```python
from build123d import *

# Parameters (mm, degrees)
SKETCH_1_W      = 20
SKETCH_1_H      = 8
EXTRUDE_1_DEPTH = 5
SKETCH_5_W      = 5
SKETCH_5_H      = 5
EXTRUDE_5_DEPTH = 10
SKETCH_8_W      = 20
SKETCH_8_H      = 8
EXTRUDE_6_DEPTH = 55
EXTRUDE_6_TAPER = 1
SKETCH_9_W      = 5
SKETCH_9_H      = 5
EXTRUDE_7_DEPTH = 11
SKETCH_10_W     = 5
SKETCH_10_H     = 5
EXTRUDE_8_DEPTH = 11


with BuildPart() as part:
    # ｽｹｯﾁ1 → ﾎﾞｽ - 押し出し1 (new body)
    with BuildSketch(Plane.XY):
        Rectangle(SKETCH_1_W, SKETCH_1_H)
    extrude(amount=EXTRUDE_1_DEPTH)

    # ｽｹｯﾁ5 → ﾎﾞｽ - 押し出し5 (add)
    with BuildSketch(Plane(origin=(0, 0, 0), x_dir=(-1, 0, 0), z_dir=(0, 0, -1))):
        Rectangle(SKETCH_5_W, SKETCH_5_H)
    extrude(amount=EXTRUDE_5_DEPTH)

    # ｽｹｯﾁ8 → ﾎﾞｽ - 押し出し6 (add)
    with BuildSketch(Plane.XY.offset(5)):
        Rectangle(SKETCH_8_W, SKETCH_8_H)
    extrude(amount=EXTRUDE_6_DEPTH, taper=EXTRUDE_6_TAPER)

    # ｽｹｯﾁ9 → ﾎﾞｽ - 押し出し7 (add)
    with BuildSketch(Plane(origin=(0, 4, 0), x_dir=(1, 0, 0), z_dir=(0, 1, 0))):
        with Locations((0, -2.5)):
            Rectangle(SKETCH_9_W, SKETCH_9_H)
    extrude(amount=EXTRUDE_7_DEPTH)

    # ｽｹｯﾁ10 → ﾎﾞｽ - 押し出し8 (add)
    with BuildSketch(Plane(origin=(0, -4, 0), x_dir=(-1, 0, 0), z_dir=(0, -1, 0))):
        with Locations((0, -2.5)):
            Rectangle(SKETCH_10_W, SKETCH_10_H)
    extrude(amount=EXTRUDE_8_DEPTH)


solid = part.part
```
Geometry check sheet. Reference: the model listing, model coordinates, mm. A direction names the side the tool comes from. Coordinates: 2 decimals unless noted, no trailing zeros. Order: outer loops, then holes, each group sorted by start corner. A loop starts at its lowest first (then second) coordinate and runs counter-clockwise, first axis right, second up.
Q1. Tool access check on faces 1 (the face through (0, 9, 5)), 2 (the face through (-2.5, -9, 3)), 3 (the face through (2.5, -9, 3)), 4 (the face through (-2.5, 0, -5)), 5 (the face through (6, 4, 2)). Record the directions out of +Z, -Z, +X, -X, +Y, -Y that give a thin tool (end or side, any length) a straight path to the whole face; none if there is none.
Reply:
face 1: +Z, +X, -X, +Y
face 2: +Z, -Z, -X, -Y
face 3: +Z, -Z, +X, -Y
face 4: -Z, -X, +Y, -Y
face 5: +Z, -Z, +X, +Y
Q2. Sectioned sample at C-C on z = 9. Record the cut outline in (x, y), and give its area (3 significant figures).
Reply:
outline: (-9.93, -3.93) - (9.93, -3.93) - (9.93, 3.93) - (-9.93, 3.93) - close
area: 156 mm2
Q3. Thickness scan on probe 1 along X at (y, z) = (-12, 1); probe 2 along Z at (x, y) = (-3.5, -1.5); probe 3 along Y at (x, z) = (4.5, 4). Record the ranges inside material, lowest first.
Reply:
probe 1: x = -2.5 to 2.5
probe 2: z = 0 to 60
probe 3: y = -4 to 4
Q4. Sectioned sample at B-B on x = -1. Record the cut outline in (y, z), and give its area (3 significant figures).
Reply:
outline: (-15, 0) - (-2.5, 0) - (-2.5, -10) - (2.5, -10) - (2.5, 0) - (15, 0) - (15, 5) - (4, 5) - (3.04, 60) - (-3.04, 60) - (-4, 5) - (-15, 5) - close
area: 587 mm2
Q5. Sectioned sample at A-A on y = 0. Record the cut outline in (x, z), and give its area (3 significant figures).
Reply:
outline: (-10, 0) - (-2.5, 0) - (-2.5, -10) - (2.5, -10) - (2.5, 0) - (10, 0) - (10, 5) - (9.04, 60) - (-9.04, 60) - (-10, 5) - close
area: 1,200 mm2
Q6. Depth check by flat-ended pin: pin 1 Ø2.5 at (x, z) = (4.5, 2.5) entering from +Y; pin 2 Ø1 at (x, z) = (2.5, 12.5) entering from +Y; pin 3 Ø6 at (y, z) = (-1, 21.5) entering from +X. Enter the tip coordinate at first touch or a pass-through.
Reply:
pin 1: stops at y = 4
pin 2: stops at y = 3.88
pin 3: stops at x = 9.76
Q7. Sectioned sample at D-D on x = 6. Record the cut outline in (y, z), and give its area (3 significant figures).
Reply:
outline: (-4, 0) - (4, 0) - (4, 5) - (3.04, 60) - (-3.04, 60) - (-4, 5) - close
area: 427 mm2
